```python
from build123d import *

# Parameters (mm, degrees)
F2_DEPTH        = 3
F4_D            = 5.5
F4_COPIES_COUNT = 3
F4_COPIES_ANGLE = 25
F5_R            = 5


# Not quite as in the source:
# - a pattern or mirror of a feature is missing from the dataset's text; its kind, count and spacing are read off the source's solid


with BuildPart() as f2:
    # F1 (on Front) → F2 (new body)
    with BuildSketch(Plane.XZ):
        with BuildLine():
            Line((604.669567257, -162.0207222342), (695.4665949281, -186.3497124738))
            ThreePointArc((695.4665949281, -186.3497124738), (720, 0), (695.4665949281, 186.3497124738))
            Line((695.4665949281, 186.3497124738), (604.669567257, 162.0207222342))
            ThreePointArc((604.669567257, 162.0207222342), (626, 0), (604.669567257, -162.0207222342))
        make_face()
    extrude(amount=-F2_DEPTH)

    # F4 (through all)
    with Locations(Plane.XZ):
        with Locations((617.0190764998, -136.7898360089)):
            f4 = Hole(F4_D / 2)

    # F4_copies: F4 ×3 about axis
    f4_copies_axis = Axis((0, 0, 0), (0, -1, 0))
    for i in range(1, F4_COPIES_COUNT):
        add(f4.rotate(f4_copies_axis, i * F4_COPIES_ANGLE / (F4_COPIES_COUNT - 1)), mode=Mode.SUBTRACT)

    # F5
    f5_edges = [f2.edges().sort_by_distance(p)[0] for p in [
        (695.466595, 1.5, 186.349712),
        (604.669567, 1.5, 162.020722),
        (695.466595, 1.5, -186.349712),
        (604.669567, 1.5, -162.020722),
    ]]
    fillet(f5_edges, radius=F5_R)


solid = f2.part
```
Work out the finished part from the listing and answer in its coordinate system (mm). Give positions to 0.01 mm unless a question says otherwise; leave off trailing zeros. Loops run counter-clockwise (first coordinate to the right, second up) from the corner with the lowest first, then second, coordinate; pieces in that order, holes last. Notation, with made-up numbers: (24, 72.5) -> (40, 72.5) arc R24 cw to (40, 103.5) -> close; hole circle Ø5 at (60.5, 69.25). An arc over 180 degrees is marked (long way). Write item = value, one per line. Start each with the question number.
(1) Given pin 1 Ø4.5 at (x, z) = (617.02, 136.79) entering from -Y; pin 2 Ø1.5 at (y, z) = (0.5, 18) entering from +X, each flat-ended and moving along its own axis, determine where each tip first touches the part or whether it passes through.
(2) Find section A-A on y = 1.05. Give the vertices of the cut face in (x, z), and give its area (3 significant figures).
(3) Find section C-C on x = 662.5. Give the vertices of the cut face in (y, z), and give its area (3 significant figures).
(4) Find the intervals of material crossed by probe 1 along X at (y, z) = (2.3, 0); probe 2 along X at (y, z) = (2.4, -135.5); probe 3 along Z at (x, y) = (632, 1.3), in increasing order. Write a range as from..to.
(5) Find section B-B on z = -48.5. Give the vertices of the cut face in (x, y), and give its area (3 significant figures).
From the geometry:
q1.pin_1 = through
q1.pin_2 = 719.79
q2.outline = (605.93, -157.22) arc R5 ccw to (609.48, -163.31) -> (690.62, -185.05) arc R5 ccw to (696.75, -181.48) arc R720 ccw to (696.75, 181.48) arc R5 ccw to (690.62, 185.05) -> (609.48, 163.31) arc R5 ccw to (605.93, 157.22) arc R626 cw to start; hole circle Ø5.5 at (617.02, -136.79); hole circle Ø5.5 at (617.02, 136.79); hole circle Ø5.5 at (632, 0)
q2.area = 33,000 mm^2
q3.outline = (0, -177.52) -> (3, -177.52) -> (3, 177.52) -> (0, 177.52) -> close
q3.area = 1,070 mm^2
q4.probe_1 = 626..629.25, 634.75..720
q4.probe_2 = 611.16..614.59, 619.45..707.13
q4.probe_3 = -169.34..-2.75, 2.75..169.34
q5.outline = (624.12, 0) -> (718.36, 0) -> (718.36, 3) -> (624.12, 3) -> close
q5.area = 283 mm^2
